from build123d import *

# Parameters (mm, degrees)
BOSS_EXTRUDE1_DEPTH            = 9.525
BOSS_EXTRUDE1_DEPTH_BACK       = 9.525
SKETCH1_R                      = 6.35
SKETCH1_R_2                    = 3.175
SKETCH2_R                      = 12.7
SKETCH2_R_2                    = 6.35
SKETCH2_R_3                    = 3.175
BOSS_EXTRUDE3_DEPTH            = 4.7625
SKETCH3_R                      = 3.175
BOSS_EXTRUDE4_DEPTH            = 28.575
FILLET1_R                      = 2.54
CHAMFER1_SIZE                  = 0.635
CUT_EXTRUDE1_DEPTH             = 13.97
CUT_EXTRUDE2_REACH             = 39.354
SKETCH6_R                      = 1.5875
CUT_EXTRUDE2_DIRECTION_2_REACH = 39.354


# Read off the part's stored shape, not the designer's step: CSK for M3 Flat Head Machine Screw1
with BuildPart() as part:
    # Sketch1 → Boss-Extrude1 (new, two sides: drawn at the far end of the back side and taken through both)
    with BuildSketch(Plane.XY.offset(-BOSS_EXTRUDE1_DEPTH_BACK)):
        Circle(SKETCH1_R)
        Circle(SKETCH1_R_2, mode=Mode.SUBTRACT)
    extrude(amount=BOSS_EXTRUDE1_DEPTH + BOSS_EXTRUDE1_DEPTH_BACK)

    # Sketch2 → Boss-Extrude3 (add)
    # profile 1 of 2: a face of its own
    with BuildSketch(Plane(origin=(0, 0, -9.525), x_dir=(-1, 0, 0), z_dir=(0, 0, -1))):
        with Locations(Location((0, 0, 0), (0, 0, 180))):
            Circle(SKETCH2_R)
        with Locations(Location((0, 0, 0), (0, 0, 180))):
            Circle(SKETCH2_R_2, mode=Mode.SUBTRACT)
    # profile 2 of 2: a face of its own
    with BuildSketch(Plane(origin=(0, 0, -9.525), x_dir=(-1, 0, 0), z_dir=(0, 0, -1))):
        with Locations(Location((0, 0, 0), (0, 0, 180))):
            Circle(SKETCH2_R_2)
        with Locations(Location((0, 0, 0), (0, 0, 180))):
            Circle(SKETCH2_R_3, mode=Mode.SUBTRACT)
    boss_extrude3 = extrude(amount=BOSS_EXTRUDE3_DEPTH)

    # Mirror1: Boss-Extrude3 across plane
    add(boss_extrude3.mirror(Plane.XY))

    # Sketch3 → Boss-Extrude4 (add, through all)
    with BuildSketch(Plane(origin=(0, 0, -14.2875), x_dir=(-1, 0, 0), z_dir=(0, 0, -1))):
        Circle(SKETCH3_R)
    extrude(amount=-BOSS_EXTRUDE4_DEPTH)

    # Fillet1
    fillet1_edges = [part.edges().sort_by_distance(p)[0] for p in [
        (-6.35, 0, -9.525),
        (-6.35, 0, 9.525),
    ]]
    fillet(fillet1_edges, radius=FILLET1_R)

    # Chamfer1
    chamfer1_edges = [part.edges().sort_by_distance(p)[0] for p in [
        (-12.7, 0, -9.525),
        (-12.7, 0, -14.2875),
        (-12.7, 0, 14.2875),
        (-12.7, 0, 9.525),
    ]]
    chamfer(chamfer1_edges, length=CHAMFER1_SIZE)

    # Sketch4 → Cut-Extrude1 (cut)
    with BuildSketch(Plane.XY.offset(14.2875)):
        with BuildLine():
            Line((1.651, 2.711977876), (-1.651, 2.711977876))
            ThreePointArc((-1.651, 2.711977876), (-1.555425987, -2.767900829), (3.175, 0))
            ThreePointArc((3.175, 0), (2.767900829, 1.555425987), (1.651, 2.711977876))
        make_face()
    extrude(amount=-CUT_EXTRUDE1_DEPTH, mode=Mode.SUBTRACT)

    # Sketch6 → Cut-Extrude2 (cut, up to next)
    with BuildSketch(Plane(origin=(-6.544693312, 1.737013471, 14.2875), x_dir=(0.9927863104442903, -0.05092138559106857, 0.1085465535330304), z_dir=(-0.11989721345558171, -0.4216449495917331, 0.8987993072368112)), mode=Mode.PRIVATE) as cut_extrude2_sk1:
        with Locations(Location((0, 0, 0), (0, 0, 75.6633116))):
            Circle(SKETCH6_R)
    cut_extrude2_tool1 = extrude(cut_extrude2_sk1.sketch, amount=-CUT_EXTRUDE2_REACH, mode=Mode.PRIVATE) & part.part
    add(cut_extrude2_tool1.solids().sort_by_distance((-6.544693, 1.737013, 14.2875))[0], mode=Mode.SUBTRACT)

    # Sketch6 → Cut-Extrude2 direction 2 (cut, up to next)
    with BuildSketch(Plane(origin=(-6.544693312, 1.737013471, 14.2875), x_dir=(0.9927863104442903, -0.05092138559106857, 0.1085465535330304), z_dir=(-0.11989721345558171, -0.4216449495917331, 0.8987993072368112)), mode=Mode.PRIVATE) as cut_extrude2_direction_2_sk1:
        with Locations(Location((0, 0, 0), (0, 0, 75.6633116))):
            Circle(SKETCH6_R)
    cut_extrude2_direction_2_tool1 = extrude(cut_extrude2_direction_2_sk1.sketch, amount=CUT_EXTRUDE2_DIRECTION_2_REACH, mode=Mode.PRIVATE) & part.part
    add(cut_extrude2_direction_2_tool1.solids().sort_by_distance((-6.544693, 1.737013, 14.2875))[0], mode=Mode.SUBTRACT)

    # CSK for M3 Flat Head Machine Screw1 outl → CSK for M3 Flat Head Machine Screw1 (revolve, cut)
    with BuildSketch(Plane(origin=(0, 0, 3.811254633), x_dir=(-0.0350043317696159, 0.9993871605926117, 0), z_dir=(0, 0, -1))):
        Polygon((0, 2.681318057), (1.7, 2.681318057), (1.7, 4.9), (3.150097206, 6.350097206), (0, 6.350097206), align=None)
    revolve(axis=Axis((0, 0, 3.811254633), (0.9993871605926117, 0.0350043317696159, 0)), mode=Mode.SUBTRACT)


solid = part.part
Verification items for the finished model (mm, model axes). A direction names the side the tool comes from. Coordinates: 2 decimals unless noted, no trailing zeros. Loops run counter-clockwise (first coordinate to the right, second up) from the corner with the lowest first, then second, coordinate; pieces in that order, holes last. Notation, with made-up numbers: M 14,83.5 L 59,83.5 A16 cw 59,87.5 Z; hole C -20.75,44 d2. An arc over 180 degrees is marked long. One line per item, written item: value.
1. Material ranges on line 1 along Z through (x, y) = (9.5, 3.5) (1 decimal); line 2 along Y through (x, z) = (0, 10.5) (3 decimals); line 3 along Z through (x, y) = (0.5, -7), recorded low to high. Write a range as from..to.
Answers follow:
line 1: -14.3..-9.5, 9.5..14.3
line 2: -12.7..-3.175, 2.712..12.7
line 3: -14.29..-8.7, 8.7..14.29
2. Gauge pin test, flat ends, axial feed: P1, Ø2, axis at x = -3.5, z = 8, coming from the +Y side; P2, Ø10, axis at x = 6.5, z = 0.5, coming from the +Y side; P3, Ø3, axis at x = 8.5, z = -8.5, coming from the +Y side; P4, Ø7.5, axis at x = 0, y = 0, coming from the +Z side. Record the tip position at first contact, or that the pin passes through.
Answers follow:
P1: y = 6.55
P2: y = 6.17
P3: y = 9.6
P4: z = 14.29
3. Set-up check for faces 5 (the flat face through (3, 3, 14.288)), 6 (the flat face through (-1, 9, 9.525)): record each of +Z, -Z, +X, -X, +Y, -Y from which the full face is reachable in a straight line by a thin tool's end or side.
Answers follow:
face 5: +Z, +X, -X, +Y, -Y
face 6: none
4. Section check B-B on z = -1. Record the cut outline in (x, y), plus the area to 3 significant figures.
Answers follow:
outline: C 0,0 d12.7
area: 127 mm^2
5. Mould release check, pull along Z, two halves, no side actions. Record for faces 1 (the flat face through (-1, 9, -9.525)), 2 (the flat face through (0, 0, 0.317)), 3 (the flat face through (0, 2.712, 7)), 4 (the cylindrical face through (-4.76, 2.35, 11.29)): pulls with the +Z half, pulls with the -Z half, needs draft (parallel to the pull), parting line crosses it, or undercut.
Answers follow:
face 1: undercut
face 2: pulls with the +Z half
face 3: needs draft
face 4: undercut
